Autodesk Inventor part; units mm, degrees
ref_plane "YZ Plane" through (0, 0, 0) normal (1, 0, 0) x (0, 1, 0)
ref_plane "XZ Plane" through (0, 0, 0) normal (0, 1, 0) x (-1, 0, 0)
ref_plane "XY Plane" through (0, 0, 0) normal (0, 0, 1) x (1, 0, 0)
sketch "Sketch1" plane through (0, 0, 0) normal (0, 0, 1) x (1, 0, 0)
  line L0 (8.0644, -32.7837) -> (-6.6856, -32.7837)
  line L1 (-6.6856, -32.7837) -> (-6.6856, -47.5337)
  line L2 (-6.6856, -47.5337) -> (8.0644, -47.5337)
  line L3 (8.0644, -47.5337) -> (8.0644, -32.7837)
  line L4 (9.5644, -31.2837) -> (-8.1856, -31.2837)
  line L5 (-8.1856, -31.2837) -> (-8.1856, -49.0337)
  line L6 (-8.1856, -49.0337) -> (9.5644, -49.0337)
  line L7 (9.5644, -49.0337) -> (9.5644, -31.2837)
  point P0 (0, 0)
  dimension "d0" = 1.5
  dimension "d1" = 1.5
  dimension "d2" = 1.5
  dimension "d3" = 1.5
  dimension "d4" = 14.75
  dimension "d5" = 14.75
extrude "Extrusion1" add sketch "Sketch1" along normal blind 4
sketch "Sketch2" plane through (-8.1856, -31.2837, 0) normal (0, 1, 0) x (1, 0, 0)
  line L0 (17.75, 0) -> (0, 0)
  line L1 (0, 0) -> (0, -4)
  line L2 (17.75, -4) -> (0, -4)
  line L3 (17.75, 0) -> (17.75, -4)
  circle A0 centre (8.75, -2) radius 2
  point P0 (8.1856, 0)
  dimension "d8" = 4
  dimension "d9" = 9
extrude "Extrusion2" add sketch "Sketch2" along normal blind 30 contours A0
properties part number "eye_cam_holder"
Read the model definition and answer for the solid it produces. Units are mm, in the model's axes. A direction names the side the tool comes from. Coordinates: 2 decimals unless noted, no trailing zeros. Write each loop counter-clockwise with the first axis right and the second up, starting at its lowest first coordinate (ties: lowest second). Pieces come first, ordered by that corner, then holes. Notation, with made-up numbers: M 29.5,48.25 L 56.5,48.25 A23 cw 56.5,72.25 Z; hole C -29,9 d11. An arc over 180 degrees is marked long. Use a Markdown table: item, result.
Q1. The part is cut by section A-A, the plane y = -44. Write down the section's boundary in (x, z), then the cut area to 3 significant figures.
Answer block:
| item | result |
|---|---|
| outline | M -8.19,0 L -6.69,0 L -6.69,4 L -8.19,4 Z; M 8.06,0 L 9.56,0 L 9.56,4 L 8.06,4 Z |
| area | 12.0 mm2 |
Q2. Straight lines are drawn through the part: L1, parallel to X at y = -45.5, z = 2.2; L2, parallel to Y at x = 4.5, z = 1.4; L3, parallel to Y at x = 0.5, z = 0.8. For each, find the intervals that lie inside material, in ascending order. Write a range as [from, to].
Answer block:
| item | result |
|---|---|
| L1 | x = [-8.19, -6.69], [8.06, 9.56] |
| L2 | y = [-49.03, -47.53], [-32.78, -31.28] |
| L3 | y = [-49.03, -47.53], [-32.78, -1.28] |
Q3. The part is cut by section D-D, the plane x = 8.75. Write down the section's boundary in (y, z).
Answer block:
| item | result |
|---|---|
| outline | M -49.03,0 L -31.28,0 L -31.28,4 L -49.03,4 Z |
Q4. Which of the six approach directions +Z, -Z, +X, -X, +Y, -Y give full straight-line access (tool end or side, diameter ignored) to faces 4 (the face through (8.064, -40, 2)), 5 (the face through (9.564, -40, 2))?
Answer block:
| item | result |
|---|---|
| face 4 | +Z, -Z |
| face 5 | +Z, -Z, +X, +Y, -Y |
Q5. Determine the mould class of faces 1 (the face through (0.131, -16.494, 0.048)), 2 (the face through (1, -49.034, 2)), 3 (the face through (1, -47.534, 2)) for opening direction X: released by +X, released by -X, zero draft, split by the parting line, or undercut.
Answer block:
| item | result |
|---|---|
| face 1 | split by the parting line |
| face 2 | zero draft |
| face 3 | undercut |
Q6. The part is cut by section C-C, the plane x = -2.75. Write down the section's boundary in (y, z), then the cut area to 3 significant figures.
Answer block:
| item | result |
|---|---|
| outline | M -49.03,0 L -47.53,0 L -47.53,4 L -49.03,4 Z; M -32.78,0 L -31.28,0 L -31.28,4 L -32.78,4 Z |
| area | 12.0 mm2 |
Q7. Each of these flat-tipped pins is pushed along its axis until it touches: pin 1 Ø2 at (x, y) = (4.5, -25) entering from -Z; pin 2 Ø1.2 at (x, z) = (7, 2.5) entering from +Y. Where does it stop, or does it pass through?
Answer block:
| item | result |
|---|---|
| pin 1 | passes through |
| pin 2 | stops at y = -31.28 |
Q8. The part is cut by section B-B, the plane z = 2. Write down the section's boundary in (x, y).
Answer block:
| item | result |
|---|---|
| outline | M -8.19,-49.03 L 9.56,-49.03 L 9.56,-31.28 L 2.56,-31.28 L 2.56,-1.28 L -1.44,-1.28 L -1.44,-31.28 L -8.19,-31.28 Z; hole M -6.69,-47.53 L 8.06,-47.53 L 8.06,-32.78 L -6.69,-32.78 Z |
